```python
from build123d import *

# Parameters (mm, degrees)
BOSS_EXTRUDE1_DEPTH     = 2
SKETCH2_R               = 2
BOSS_EXTRUDE2_DEPTH     = 8
CROQUIS1_R              = 0.75
CORTAR_EXTRUIR1_DEPTH   = 10
CORTAR_EXTRUIR2_START   = -16
CROQUIS2_R              = 2
CORTAR_EXTRUIR2_DEPTH   = 16
SALIENTE_EXTRUIR1_START = -2
CROQUIS3_R              = 3.5
CROQUIS3_R_2            = 2
SALIENTE_EXTRUIR1_DEPTH = 2


with BuildPart() as part:
    # Sketch1 → Boss-Extrude1 (new body)
    with BuildSketch(Plane.XY):
        with BuildLine():
            Line((0, -2), (40, -2))
            ThreePointArc((40, -2), (42, 0), (40, 2))
            Line((40, 2), (0, 2))
            ThreePointArc((0, 2), (-2, 0), (0, -2))
        make_face()
    extrude(amount=BOSS_EXTRUDE1_DEPTH)

    # Sketch2 → Boss-Extrude2 (add)
    with BuildSketch(Plane.XY.offset(2)):
        with Locations(Location((0, 0, 0), (0, 0, 270))):
            Circle(SKETCH2_R)
    extrude(amount=BOSS_EXTRUDE2_DEPTH)

    # Croquis1 → Cortar-Extruir1 (cut)
    with BuildSketch(Plane.XY.offset(2)):
        with Locations((40, 0)):
            Circle(CROQUIS1_R)
    extrude(amount=-CORTAR_EXTRUIR1_DEPTH, mode=Mode.SUBTRACT)

    # Croquis2 → Cortar-Extruir2 (cut)
    with BuildSketch(Plane.XY.offset(10).offset(CORTAR_EXTRUIR2_START)):
        Circle(CROQUIS2_R)
    extrude(amount=CORTAR_EXTRUIR2_DEPTH, mode=Mode.SUBTRACT)

    # Croquis3 → Saliente-Extruir1 (add)
    with BuildSketch(Plane.XY.offset(2).offset(SALIENTE_EXTRUIR1_START)):
        Circle(CROQUIS3_R)
        Circle(CROQUIS3_R_2, mode=Mode.SUBTRACT)
    extrude(amount=SALIENTE_EXTRUIR1_DEPTH)


solid = part.part
```
For this review, take the finished solid that the model builds, in its own axes (mm). A direction names the side the tool comes from. Coordinates: 2 decimals unless noted, no trailing zeros. Write each loop counter-clockwise with the first axis right and the second up, starting at its lowest first coordinate (ties: lowest second). Pieces come first, ordered by that corner, then holes. Notation, with made-up numbers: (0.5, 43) -> (34.5, 43) arc R22 ccw to (34.5, 82) -> close; hole circle Ø3 at (-1, 74). An arc over 180 degrees is marked (long way). Put each result on its own line as item: value.
Q1. Tool access review of faces 1 (the flat face through (22, 2, 1)), 2 (the flat face through (21, -2, 1)), 3 (the flat face through (19, 0, 2)): name each direction out of +Z, -Z, +X, -X, +Y, -Y from which nothing blocks a thin tool from reaching the whole face with its end or side.
From the geometry:
face 1: +Z, -Z, +X, +Y
face 2: +Z, -Z, +X, -Y
face 3: +Z, +X, -X, +Y, -Y
Q2. Wall thickness on L1, parallel to Y at x = 0, z = 0.8; L2, parallel to X at y = -0.5, z = 1.5; L3, parallel to Y at x = 40, z = 1.05: over which ranges is each line inside the solid? List them lowest first.
From the geometry:
L1: y = -3.5 to -2, 2 to 3.5
L2: x = -3.46 to -1.94, 1.94 to 39.44, 40.56 to 41.94
L3: y = -2 to -0.75, 0.75 to 2
Q3. Take a section at B-B, the plane z = 0.35. State the section outline as (x, y) points, then the cut area to 3 significant figures.
From the geometry:
outline: (2.87, -2) -> (40, -2) arc R2 ccw to (40, 2) -> (2.87, 2) arc R3.5 ccw (long way) to start; hole circle Ø4 at (0, 0); hole circle Ø1.5 at (40, 0)
area: 177 mm2
Q4. The part is to be moulded in two halves that separate along X. For faces 4 (the cylindrical face through (40.715, 0.225, 1.014)), 5 (the cylindrical face through (2, 0, 1)), 6 (the flat face through (19, 0, 0)), 7 (the cylindrical face through (42, 0, 1)), say which applies: +X half, -X half, draft (parallel to the pull), parting line (faces both ways), or undercut.
From the geometry:
face 4: undercut
face 5: undercut
face 6: draft
face 7: +X half
Q5. Take a section at D-D, the plane x = 28. State the section outline as (y, z) points, then the cut area to 3 significant figures.
From the geometry:
outline: (-2, 0) -> (2, 0) -> (2, 2) -> (-2, 2) -> close
area: 8.00 mm2
Q6. Clearance check with a flat-ended pin moving along its axis: pin 1 Ø2.5 at (x, y) = (0, 0) entering from -Z. State where the tip first meets the part, or that it passes through.
From the geometry:
pin 1: passes through
Q7. Take a section at C-C, the plane y = 0. State the section outline as (x, z) points, then the cut area to 3 significant figures.
From the geometry:
outline: (-3.5, 0) -> (-2, 0) -> (-2, 2) -> (-3.5, 2) -> close; (2, 0) -> (39.25, 0) -> (39.25, 2) -> (2, 2) -> close; (40.75, 0) -> (42, 0) -> (42, 2) -> (40.75, 2) -> close
area: 80.0 mm2
Q8. Take a section at A-A, the plane x = 0. State the section outline as (y, z) points, then the cut area to 3 significant figures.
From the geometry:
outline: (-3.5, 0) -> (-2, 0) -> (-2, 2) -> (-3.5, 2) -> close; (2, 0) -> (3.5, 0) -> (3.5, 2) -> (2, 2) -> close
area: 6.00 mm2
